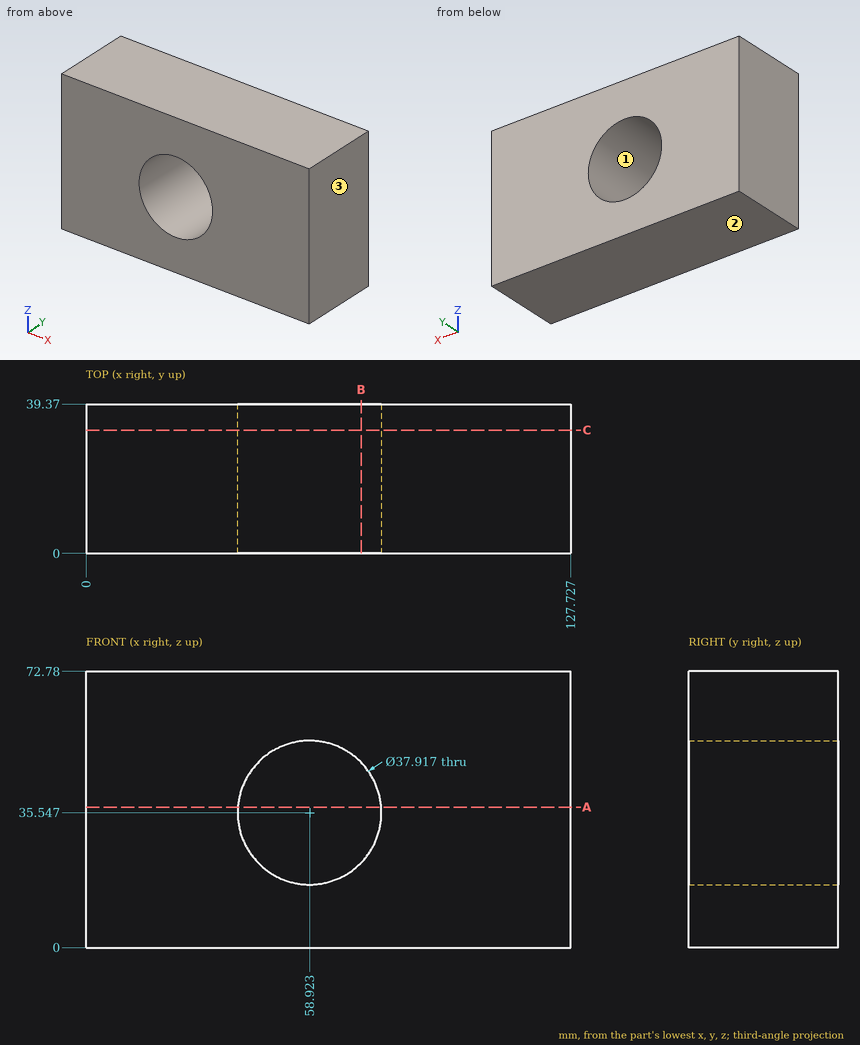
The figure shows three views and two pictorial views of one solid part (mm, origin at its lowest corner). Answer the questions. Give positions to 0.01 mm unless a question says otherwise; leave off trailing zeros. Write each loop counter-clockwise with the first axis right and the second up, starting at its lowest first coordinate (ties: lowest second). Pieces come first, ordered by that corner, then holes. Notation, with made-up numbers: M -17.75,-17 L -10.75,-17 A30 cw -10.75,17 Z; hole C -3.5,88.25 d9. An arc over 180 degrees is marked long. Write each question's results on one line, items separated by ' | '.
Q1. For a pull along Z with two mould halves and no side action, classify the marked faces 1, 2 and 3 as released by +Z, released by -Z, zero draft, split by the parting line, or undercut.
Output values:
face 1: undercut | face 2: released by -Z | face 3: zero draft
Q2. Consider L1, parallel to X at y = 18, z = 52 (1 decimal); L2, parallel to Z at x = 54, y = 29.5 (1 decimal); L3, parallel to X at y = 20, z = 33. Determine where each line is inside the solid, lowest interval first. Write a range as from..to.
Output values:
L1: 0..49.5, 68.3..127.7 | L2: 0..17.2, 53.9..72.8 | L3: 0..40.14, 77.71..127.73
Q3. Section B-B, the plane x = 72.5 is taken. Write down the section's boundary in (y, z) (1 decimal), then the cut area to 3 significant figures.
Output values:
outline: M 0,0 L 39.4,0 L 39.4,22.3 L 0,22.3 Z; M 0,48.8 L 39.4,48.8 L 39.4,72.8 L 0,72.8 Z | area: 1,820 mm2
Q4. Section C-C, the plane y = 32.5 is taken. Write down the section's boundary in (x, z).
Output values:
outline: M 0,0 L 127.73,0 L 127.73,72.78 L 0,72.78 Z; hole C 58.92,35.55 d37.92
Q5. Section A-A, the plane z = 37 is taken. Write down the section's boundary in (x, y) (1 decimal), then the cut area to 3 significant figures.
Output values:
outline: M 0,0 L 40,0 L 40,39.4 L 0,39.4 Z; M 77.8,0 L 127.7,0 L 127.7,39.4 L 77.8,39.4 Z | area: 3,540 mm2
